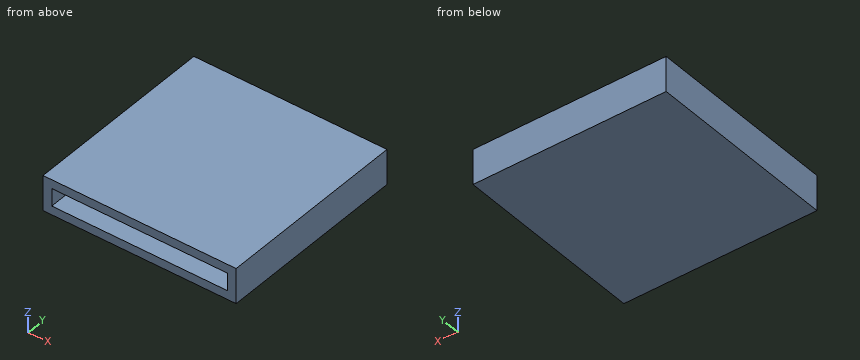
from build123d import *

# Parameters (mm, degrees)
F0_W     = 12.7
F0_H     = 266.7
F1_DEPTH = 50.8
F2_W     = 254
F2_H     = 12.7
F3_DEPTH = 266.7
F4_W     = 254
F4_H     = 12.7
F5_DEPTH = 266.7


with BuildPart() as f1:
    # F0 (on Top) → F1 (new body)
    with BuildSketch(Plane.XY):
        Polygon((-127, 139.7), (-139.7, 139.7), (-139.7, -139.7), (-127, -139.7), (-127, 127), align=None)
        Polygon((139.7, 139.7), (-127, 139.7), (-127, 127), (127, 127), (139.7, 127), align=None)
        with Locations((133.35, -6.35)):
            Rectangle(F0_W, F0_H)
    extrude(amount=F1_DEPTH)

    # F2 (on face) → F3 (join)
    with BuildSketch(Plane.XZ.offset(-127)):
        with Locations((0, 44.45)):
            Rectangle(F2_W, F2_H)
    extrude(amount=F3_DEPTH)

    # F4 (on face) → F5 (join)
    with BuildSketch(Plane.XZ.offset(-127)):
        with Locations((0, 6.35)):
            Rectangle(F4_W, F4_H)
    extrude(amount=F5_DEPTH)


solid = f1.part
Verification items for the finished model (mm, model axes). Give positions to 0.01 mm unless a question says otherwise; leave off trailing zeros. Write each loop counter-clockwise with the first axis right and the second up, starting at its lowest first coordinate (ties: lowest second). Pieces come first, ordered by that corner, then holes.
(1) Material ranges on line 1 (X direction, y = -32.5, z = 28.5); line 2 (Z direction, x = 46, y = 61); line 3 (Y direction, x = 50, z = 35.5), recorded low to high.
(2) Cross-section at A-A (y = -56). Enter the section's corners in (x, z), plus the area to 3 significant figures.
(3) Gauge pin test, flat end, axial feed: pin 1 (20.5 mm diameter, centred on x = -25, z = 19.5, fed in from -Y). Record the tip position at first contact, or that the pin passes through.
(4) Cross-section at C-C (z = 26.5). Enter the section's corners in (x, y).
(5) Cross-section at B-B (x = 0). Enter the section's corners in (y, z), plus the area to 3 significant figures.
Worked out:
1. line 1: x = -139.7 to -127, 127 to 139.7
1. line 2: z = 0 to 12.7, 38.1 to 50.8
1. line 3: y = 127 to 139.7
2. outline: (-139.7, 0) - (139.7, 0) - (139.7, 50.8) - (-139.7, 50.8) - close; hole (-127, 12.7) - (127, 12.7) - (127, 38.1) - (-127, 38.1) - close
2. area: 7,740 mm2
3. pin 1: stops at y = -139.7
4. outline: (-139.7, -139.7) - (-127, -139.7) - (-127, 127) - (127, 127) - (127, -139.7) - (139.7, -139.7) - (139.7, 139.7) - (-139.7, 139.7) - close
5. outline: (-139.7, 0) - (139.7, 0) - (139.7, 50.8) - (-139.7, 50.8) - (-139.7, 38.1) - (127, 38.1) - (127, 12.7) - (-139.7, 12.7) - close
5. area: 7,420 mm2
